The model under review builds one solid part; all positions refer to its coordinate system, in mm. Face numbers are marked on the shaded views. A direction names the side the tool comes from. Give positions to 0.01 mm unless a question says otherwise; leave off trailing zeros. Loops run counter-clockwise (first coordinate to the right, second up) from the corner with the lowest first, then second, coordinate; pieces in that order, holes last. Notation, with made-up numbers: M 52,37 L 60,37 A19 cw 60,68 Z; hole C 69.5,-0.5 d6. An arc over 180 degrees is marked long. Return JSON: item names as keys, results as strings.
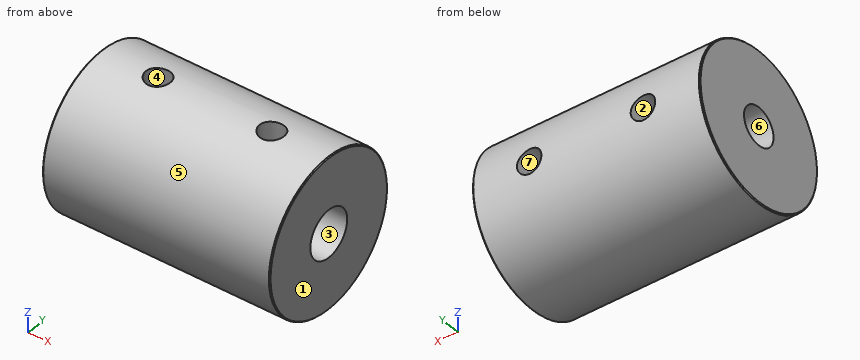
```python
from build123d import *

# Parameters (mm, degrees)
SKETCH_1_R               = 8
EXTRUDE_1_DEPTH          = 24
SKETCH_2_R               = 2
CUT_EXTRUDE_1_DEPTH      = 12
SKETCH_3_R               = 2.5
CUT_EXTRUDE_2_DEPTH      = 12
CUT_EXTRUDE_3_REACH      = 28.533
CUT_EXTRUDE_3_END_RADIUS = 8
SKETCH_4_R               = 1.29
CUT_EXTRUDE_4_REACH      = 28.533
CUT_EXTRUDE_4_END_RADIUS = 8
SKETCH_5_R               = 1.29
CHAMFER_1_SIZE           = 0.1


with BuildPart() as part:
    # 草图1 → 凸台-拉伸1 (new body)
    with BuildSketch(Plane(origin=(0, 0, 0), x_dir=(0, 0, -1), z_dir=(1, 0, 0))):
        Circle(SKETCH_1_R)
    extrude(amount=EXTRUDE_1_DEPTH)

    # 草图2 → 切除-拉伸1 (cut)
    with BuildSketch(Plane.ZY):
        Circle(SKETCH_2_R)
    extrude(amount=-CUT_EXTRUDE_1_DEPTH, mode=Mode.SUBTRACT)

    # 草图3 → 切除-拉伸2 (cut)
    with BuildSketch(Plane(origin=(24, 0, 0), x_dir=(0, 0, -1), z_dir=(1, 0, 0))):
        Circle(SKETCH_3_R)
    extrude(amount=-CUT_EXTRUDE_2_DEPTH, mode=Mode.SUBTRACT)

    # 切除-拉伸3: up to this cylinder (the profile starts inside it)
    cut_extrude_3_end = Plane(origin=(12, 0, 0), z_dir=(-1, 0, 0)) * Cylinder(CUT_EXTRUDE_3_END_RADIUS, 86.066, mode=Mode.PRIVATE)
    # 草图4 → 切除-拉伸3 (cut, up to the surface)
    with BuildSketch(Plane(origin=(0, 0, 0), x_dir=(1, 0, 0), z_dir=(0, 1, 0)), mode=Mode.PRIVATE) as cut_extrude_3_sk1:
        with Locations(Location((6, 0, 0), (0, 0, 90))):
            Circle(SKETCH_4_R)
    cut_extrude_3_tool1 = extrude(cut_extrude_3_sk1.sketch, amount=CUT_EXTRUDE_3_REACH, mode=Mode.PRIVATE) & cut_extrude_3_end
    add(cut_extrude_3_tool1.solids().sort_by_distance((6, 0, 0))[0], mode=Mode.SUBTRACT)
    # 草图4 → 切除-拉伸3 (cut, up to the surface)
    with BuildSketch(Plane(origin=(0, 0, 0), x_dir=(1, 0, 0), z_dir=(0, 1, 0)), mode=Mode.PRIVATE) as cut_extrude_3_sk2:
        with Locations(Location((18, 0, 0), (0, 0, 90))):
            Circle(SKETCH_4_R)
    cut_extrude_3_tool2 = extrude(cut_extrude_3_sk2.sketch, amount=CUT_EXTRUDE_3_REACH, mode=Mode.PRIVATE) & cut_extrude_3_end
    add(cut_extrude_3_tool2.solids().sort_by_distance((18, 0, 0))[0], mode=Mode.SUBTRACT)

    # 切除-拉伸4: up to this cylinder (the profile starts inside it)
    cut_extrude_4_end = Plane(origin=(12, 0, 0), z_dir=(-1, 0, 0)) * Cylinder(CUT_EXTRUDE_4_END_RADIUS, 86.066, mode=Mode.PRIVATE)
    # 草图5 → 切除-拉伸4 (cut, up to the surface)
    with BuildSketch(Plane.XY, mode=Mode.PRIVATE) as cut_extrude_4_sk1:
        with Locations(Location((18, 0, 0), (0, 0, 180))):
            Circle(SKETCH_5_R)
    cut_extrude_4_tool1 = extrude(cut_extrude_4_sk1.sketch, amount=CUT_EXTRUDE_4_REACH, mode=Mode.PRIVATE) & cut_extrude_4_end
    add(cut_extrude_4_tool1.solids().sort_by_distance((18, 0, 0))[0], mode=Mode.SUBTRACT)
    # 草图5 → 切除-拉伸4 (cut, up to the surface)
    with BuildSketch(Plane.XY, mode=Mode.PRIVATE) as cut_extrude_4_sk2:
        with Locations(Location((6, 0, 0), (0, 0, 180))):
            Circle(SKETCH_5_R)
    cut_extrude_4_tool2 = extrude(cut_extrude_4_sk2.sketch, amount=CUT_EXTRUDE_4_REACH, mode=Mode.PRIVATE) & cut_extrude_4_end
    add(cut_extrude_4_tool2.solids().sort_by_distance((6, 0, 0))[0], mode=Mode.SUBTRACT)

    # 倒角1
    chamfer_1_edges = [part.edges().sort_by_distance(p)[0] for p in [
        (0, 0, 8),
        (24, 0, 8),
    ]]
    chamfer(chamfer_1_edges, length=CHAMFER_1_SIZE)


solid = part.part
```
1) Consider section A-A on z = 0. Write out the cut boundary in (x, y), then the cut area to 3 significant figures.
From the geometry:
{"outline": "M 0,-7.9 L 0.1,-8 L 23.9,-8 L 24,-7.9 L 24,-2.5 L 12,-2.5 L 12,-2 L 0,-2 Z; M 0,2 L 4.71,2 L 4.71,8 L 0.1,8 L 0,7.9 Z; M 7.29,2 L 12,2 L 12,2.5 L 16.71,2.5 L 16.71,8 L 7.29,8 Z; M 19.29,2.5 L 24,2.5 L 24,7.9 L 23.9,8 L 19.29,8 Z", "area": "246 mm²"}
2) The part is to be moulded in two halves that separate along Y. For the marked faces 5, 6 and 7, say which applies: released by +Y, released by -Y, zero draft, split by the parting line, or undercut.
From the geometry:
{"face 5": "split by the parting line", "face 6": "undercut", "face 7": "zero draft"}
3) Wall thickness on L1, parallel to X at y = 4.25, z = 0; L2, parallel to Z at x = 20.75, y = 0; L3, parallel to X at y = -1, z = 7: over which ranges is each line inside the solid? List them lowest first. Write a range as from..to.
From the geometry:
{"L1": "0..4.71, 7.29..16.71, 19.29..24", "L2": "-8..-2.5, 2.5..8", "L3": "0..5.19, 6.81..17.19, 18.81..24"}
4) Consider section C-C on x = 19. Write out the cut boundary in (y, z).
From the geometry:
{"outline": "M -0.81,2.36 L -0.81,7.96 A8 ccw long 7.96,-0.81 L 2.36,-0.81 A2.5 cw long Z; M 0.81,2.36 A2.5 cw 2.36,0.81 L 7.96,0.81 A8 ccw 0.81,7.96 Z"}
5) Insertion check: pin 1 (8 mm diameter, centred on x = 20, y = 6, fed in from +Z); pin 2 (2 mm diameter, centred on x = 6, z = 0, fed in from +Y); pin 3 (2.5 mm diameter, centred on y = 0, z = 0, fed in from +X). Each pin has a flat end and moves straight along its axis. Give the tip position at first contact, or say it passes through.
From the geometry:
{"pin 1": "z = 7.75", "pin 2": "y = -1.73", "pin 3": "through"}
6) Tool access review of the marked faces 1, 2, 3 and 4: name each direction out of +Z, -Z, +X, -X, +Y, -Y from which nothing blocks a thin tool from reaching the whole face with its end or side.
From the geometry:
{"face 1": "+Z, -Z, +X, +Y, -Y", "face 2": "+Y", "face 3": "+X", "face 4": "+Z"}
7) Consider section D-D on x = 3. Write out the cut boundary in (y, z).
From the geometry:
{"outline": "C 0,0 d16; hole C 0,0 d4"}
